Can you work these out from the model? Positions are in its coordinate system, mm. A direction names the side the tool comes from. Give positions to 0.01 mm unless a question says otherwise; leave off trailing zeros. Loops run counter-clockwise (first coordinate to the right, second up) from the corner with the lowest first, then second, coordinate; pieces in that order, holes last. Notation, with made-up numbers: (0, 80) - (36, 80) arc R33 ccw to (36, 109) - close; hole circle Ø9 at (86, 33.25). An arc over 180 degrees is marked (long way). Write item = value, one per line.
from build123d import *

# Parameters (mm, degrees)
SKETCH1_R               = 20
BOSS_EXTRUDE1_DEPTH     = 22.5
SKETCH3_W               = 17.5
SKETCH3_H               = 17.5
BOSS_EXTRUDE2_DEPTH     = 18
CUT_EXTRUDE1_DEPTH      = 76.039156445
CUT_EXTRUDE1_DEPTH_BACK = 76.039156445
SKETCH4_R               = 2.75
BOSS_EXTRUDE3_DEPTH     = 66.5
SKETCH6_R               = 19.25
BOSS_EXTRUDE4_DEPTH     = 77.5
SKETCH7_R               = 10
BOSS_EXTRUDE5_DEPTH     = 30.5


with BuildPart() as part:
    # Sketch1 → Boss-Extrude1 (new body)
    with BuildSketch(Plane(origin=(0, 0, 0), x_dir=(0, 0, -1), z_dir=(1, 0, 0))):
        with Locations((0, 36.25)):
            Circle(SKETCH1_R)
        with BuildLine():
            ThreePointArc((20, 36.25), (0, 16.25), (-20, 36.25))
            Line((-20, 36.25), (-20, -12.25))
            Line((-20, -12.25), (-13.5, -18.75))
            Line((-13.5, -18.75), (13.5, -18.75))
            Line((13.5, -18.75), (20, -12.25))
            Line((20, -12.25), (20, 36.25))
        make_face()
    extrude(amount=BOSS_EXTRUDE1_DEPTH)

    # Sketch3 → Boss-Extrude2 (add)
    with BuildSketch(Plane(origin=(22.5, 0, 0), x_dir=(0, 0, -1), z_dir=(1, 0, 0))):
        Rectangle(SKETCH3_W, SKETCH3_H)
    extrude(amount=BOSS_EXTRUDE2_DEPTH)

    # Sketch4 → Cut-Extrude1 (cut, two sides: drawn at the far end of the back side and taken through both)
    with BuildSketch(Plane.XY.offset(8.75).offset(-CUT_EXTRUDE1_DEPTH_BACK)):
        with Locations(Location((33.5, 0, 0), (0, 0, 90))):
            Circle(SKETCH4_R)
    extrude(amount=CUT_EXTRUDE1_DEPTH + CUT_EXTRUDE1_DEPTH_BACK, mode=Mode.SUBTRACT)

    # Sketch5 → Boss-Extrude3 (add)
    with BuildSketch(Plane.ZY):
        with BuildLine():
            Line((-12, -18.75), (12, -18.75))
            Line((12, -18.75), (14.783645942, -2.538466597))
            ThreePointArc((14.783645942, -2.538466597), (0, 15), (-14.783645942, -2.538466597))
            Line((-14.783645942, -2.538466597), (-12, -18.75))
        make_face()
    extrude(amount=BOSS_EXTRUDE3_DEPTH)

    # Sketch6 → Boss-Extrude4 (add)
    with BuildSketch(Plane.ZY):
        with Locations(Location((0, 36.25, 0), (0, 0, 180))):
            Circle(SKETCH6_R)
    extrude(amount=BOSS_EXTRUDE4_DEPTH)

    # Sketch7 → Boss-Extrude5 (add)
    with BuildSketch(Plane.ZY.offset(66.5)):
        with Locations(Location((0, 0, 0), (0, 0, 180))):
            Circle(SKETCH7_R)
    extrude(amount=BOSS_EXTRUDE5_DEPTH)


solid = part.part
Q1. I need wall thicknesses on L1, parallel to X at y = 0, z = 0.5; L2, parallel to Y at x = 33, z = -4; L3, parallel to X at y = 34, z = -4.5. Which ranges of each line are inside material? Lowest first, please.
Output:
L1 = -97 to 30.75, 36.25 to 40.5
L2 = -8.75 to -2.7, 2.7 to 8.75
L3 = -77.5 to 22.5
Q2. Which directions (+Z, -Z, +X, -X, +Y, -Y) give clear straight access to the entire face, cutting with the end or side of a thin tool? Please do faces 5 (the flat face through (31, 8.75, 0)), 6 (the flat face through (11.09, -15.45, 16.8)), 7 (the cylindrical face through (-82, 0, 10)), 8 (the flat face through (29, 0, -8.75)), 9 (the cylindrical face through (11.092, 56.245, -0.44)).
Output:
face_5 = +Z, -Z, +X, +Y
face_6 = +Z, +X, -X, -Y
face_7 = -X
face_8 = -Z, +X, +Y, -Y
face_9 = +X, -X, +Y
Q3. Imagine slicing it at A-A, the plane y = 0. Write out the boundary of the cut face in (x, z).
Output:
outline = (-97, -10) - (-66.5, -10) - (-66.5, -15) - (0, -15) - (0, -20) - (22.5, -20) - (22.5, -8.75) - (30.75, -8.75) - (30.75, 8.75) - (22.5, 8.75) - (22.5, 20) - (0, 20) - (0, 15) - (-66.5, 15) - (-66.5, 10) - (-97, 10) - close; (36.25, -8.75) - (40.5, -8.75) - (40.5, 8.75) - (36.25, 8.75) - close
Q4. Imagine slicing it at D-D, the plane y = 12. Write out the boundary of the cut face in (x, z), then the cut area to 3 significant figures.
Output:
outline = (-66.5, -9) - (0, -9) - (0, -20) - (22.5, -20) - (22.5, 20) - (0, 20) - (0, 9) - (-66.5, 9) - close
area = 2,100 mm2
Q5. Imagine slicing it at B-B, the plane x = 33.5. Write out the boundary of the cut face in (y, z).
Output:
outline = (-8.75, -8.75) - (-2.75, -8.75) - (-2.75, 8.75) - (-8.75, 8.75) - close; (2.75, -8.75) - (8.75, -8.75) - (8.75, 8.75) - (2.75, 8.75) - close
Q6. Imagine slicing it at C-C, the plane z = 0. Write out the boundary of the cut face in (x, y).
Output:
outline = (-97, -10) - (-66.5, -10) - (-66.5, -18.75) - (22.5, -18.75) - (22.5, -8.75) - (40.5, -8.75) - (40.5, 8.75) - (22.5, 8.75) - (22.5, 56.25) - (0, 56.25) - (0, 55.5) - (-77.5, 55.5) - (-77.5, 17) - (0, 17) - (0, 15) - (-66.5, 15) - (-66.5, 10) - (-97, 10) - close; hole circle Ø5.5 at (33.5, 0)
Q7. For pin 1 (14 mm diameter, centred on x = 33, z = 1, fed in from +Y); pin 2 (3 mm diameter, centred on x = -48.5, y = 17, fed in from +Z); pin 3 (1 mm diameter, centred on x = -75.5, y = -2, fed in from -Z); pin 4 (4.5 mm diameter, centred on x = 33.5, y = 0, fed in from -Z), each with a flat end and sliding along its axis, tell me the tip position at first contact or that it passes through.
Output:
pin_1 = 8.75
pin_2 = 7.45
pin_3 = -9.89
pin_4 = through
Q8. We'd pull the mould along Y, two halves only. Please class faces 1 (the flat face through (-66.5, -9, -7)), 2 (the flat face through (0, 16, 0)), 3 (the flat face through (-77.5, 36, 0)), 4 (the flat face through (-32.78, -10.76, 13.37)): released by +Y, released by -Y, zero draft, split by the parting line, or undercut.
Output:
face_1 = undercut
face_2 = undercut
face_3 = zero draft
face_4 = released by -Y
